from build123d import *

# Parameters (mm, degrees)
BOSS_EXTRUDE1_DEPTH  = 5
SKETCH2_R            = 1.75
CUT_EXTRUDE1_DEPTH   = 66.019227925
SKETCH5_R            = 18
BOSS_EXTRUDE2_DEPTH  = 5
FILLET1_R            = 2
FILLET1_OF_MIRROR3_R = 2
SKETCH6_R            = 3.25
CUT_EXTRUDE3_DEPTH   = 4
CHAMFER1_SIZE        = 0.5


with BuildPart() as part:
    # Sketch1 → Boss-Extrude1 (new body)
    with BuildSketch(Plane(origin=(0, 0, 0), x_dir=(1, 0, 0), z_dir=(0, 1, 0))):
        with BuildLine():
            Line((-20.5, 56.5), (-20.5, -15))
            ThreePointArc((-20.5, -15), (-19.035533906, -18.535533906), (-15.5, -20))
            Line((-15.5, -20), (15.5, -20))
            ThreePointArc((15.5, -20), (19.035533906, -18.535533906), (20.5, -15))
            Line((20.5, -15), (20.5, 56.5))
            ThreePointArc((20.5, 56.5), (19.035533906, 60.035533906), (15.5, 61.5))
            Line((15.5, 61.5), (-15.5, 61.5))
            ThreePointArc((-15.5, 61.5), (-19.035533906, 60.035533906), (-20.5, 56.5))
        make_face()
    extrude(amount=-BOSS_EXTRUDE1_DEPTH)

    # Sketch2 → Cut-Extrude1 (cut, symmetric)
    with BuildSketch(Plane.XZ.offset(5)):
        with Locations(Location((-16, -57.5, 0), (0, 0, 270))):
            Circle(SKETCH2_R)
        with Locations(Location((-16, 15.5, 0), (0, 0, 270))):
            Circle(SKETCH2_R)
    cut_extrude1 = extrude(amount=CUT_EXTRUDE1_DEPTH, both=True, mode=Mode.SUBTRACT)

    # Mirror1: Cut-Extrude1 across plane
    add(cut_extrude1.mirror(Plane(origin=(0, 0, 0), x_dir=(0, 0, 1), z_dir=(1, 0, 0))), mode=Mode.SUBTRACT)

    # Sketch5 → Boss-Extrude2 (add)
    with BuildSketch(Plane(origin=(0, 0, 0), x_dir=(1, 0, 0), z_dir=(0, 1, 0))):
        with Locations(Location((0, 41.5, 0), (0, 0, 90))):
            Circle(SKETCH5_R)
    boss_extrude2 = extrude(amount=BOSS_EXTRUDE2_DEPTH)

    # Fillet1
    fillet1_edges = [part.edges().sort_by_distance(p)[0] for p in [
        (0, 5, -23.5),
    ]]
    fillet(fillet1_edges, radius=FILLET1_R)

    # Mirror3: Boss-Extrude2 across plane
    add(boss_extrude2.mirror(Plane(origin=(0, 0, -20.75), x_dir=(1, 0, 0), z_dir=(0, 0, -1))))

    # Fillet1 of Mirror3
    fillet1_of_mirror3_edges = [part.edges().sort_by_distance(p)[0] for p in [
        (0, 5, -18),
    ]]
    fillet(fillet1_of_mirror3_edges, radius=FILLET1_OF_MIRROR3_R)

    # Sketch6 → Cut-Extrude3 (cut)
    with BuildSketch(Plane.XZ.offset(5)):
        with Locations(Location((-16, -57.5, 0), (0, 0, 270))):
            Circle(SKETCH6_R)
        with Locations(Location((16, 15.5, 0), (0, 0, 270))):
            Circle(SKETCH6_R)
        with Locations(Location((-16, 15.5, 0), (0, 0, 270))):
            Circle(SKETCH6_R)
        with Locations(Location((16, -57.5, 0), (0, 0, 270))):
            Circle(SKETCH6_R)
    extrude(amount=-CUT_EXTRUDE3_DEPTH, mode=Mode.SUBTRACT)

    # Chamfer1
    chamfer1_edges = [part.edges().sort_by_distance(p)[0] for p in [
        (-19.035533906, -5, 18.535533906),
        (0, -5, 20),
        (19.035533906, -5, 18.535533906),
        (20.5, -5, -20.75),
        (19.035533906, -5, -60.035533906),
        (0, -5, -61.5),
        (-19.035533906, -5, -60.035533906),
        (-20.5, -5, -20.75),
    ]]
    chamfer(chamfer1_edges, length=CHAMFER1_SIZE)


solid = part.part
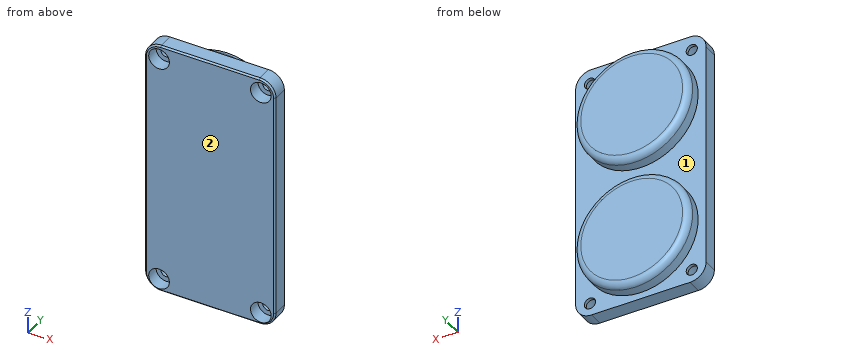
Model file for the job. Use its own axes, mm. Face numbers are marked on the shaded views. Coordinates: 2 decimals unless noted, no trailing zeros. Write each loop counter-clockwise with the first axis right and the second up, starting at its lowest first coordinate (ties: lowest second). Pieces come first, ordered by that corner, then holes. Notation, with made-up numbers: (24.5, -18.5) - (52.5, -18.5) arc R4 ccw to (52.5, -13.5) - close; hole circle Ø5 at (83.25, 79). An arc over 180 degrees is marked (long way). Write each question's results on one line, items separated by ' | '. Start each with the question number.
1) Probe line 1 along X through (y, z) = (-0.4, -57.5); line 2 along X through (y, z) = (-2.2, 15.5); line 3 along Y through (x, z) = (-17, -7.5). List the from-to ranges inside material, lowest first. Write a range as from..to.
2) Flat gauge pins, fed straight in: P1, Ø4, axis at x = 16, z = -57.5, coming from the +Y side; P2, Ø2, axis at x = -17, z = -58, coming from the -Y side; P3, Ø2, axis at x = -16, z = 15.5, coming from the -Y side; P4, Ø4, axis at y = 3.5, z = -30.5, coming from the +X side. Where does each tip first touch, or does it go through?
3) Cut at C-C (y = 1.5). Write the cut outline in (x, z).
4) Cut at B-B (x = 0). Write the cut outline in (y, z), then the cut area to 3 significant figures.
5) Cut at A-A (y = -3.25). Write the cut outline in (x, z), then the cut area to 3 significant figures.
6) Mould opens along Z. For the marked faces 1 and 2 say: pulls with the +Z half, pulls with the -Z half, needs draft (parallel to the pull), parting line crosses it, or undercut.
Returned:
1) line 1: -20.4..-17.75, -14.25..14.25, 17.75..20.4 | line 2: -20.47..-19.25, -12.75..12.75, 19.25..20.47 | line 3: -5..0
2) P1: y = 0 | P2: y = -1 | P3: through | P4: x = 15.56
3) outline: circle Ø36 at (0, -41.5); circle Ø36 at (0, 0)
4) outline: (-5, -61) - (-4.5, -61.5) - (0, -61.5) - (0, -59.5) - (3, -59.5) arc R2 ccw to (5, -57.5) - (5, -25.5) arc R2 ccw to (3, -23.5) - (0, -23.5) - (0, -18) - (3, -18) arc R2 ccw to (5, -16) - (5, 16) arc R2 ccw to (3, 18) - (0, 18) - (0, 20) - (-4.5, 20) - (-5, 19.5) - close | area: 764 mm^2
5) outline: (-20.5, -56.5) arc R5 ccw to (-15.5, -61.5) - (15.5, -61.5) arc R5 ccw to (20.5, -56.5) - (20.5, 15) arc R5 ccw to (15.5, 20) - (-15.5, 20) arc R5 ccw to (-20.5, 15) - close; hole circle Ø6.5 at (-16, -57.5); hole circle Ø6.5 at (-16, 15.5); hole circle Ø6.5 at (16, -57.5); hole circle Ø6.5 at (16, 15.5) | area: 3,190 mm^2
6) face 1: undercut | face 2: needs draft
